Read the model definition and answer for the solid it produces. Units are mm, in the model's axes. Face numbers are marked on the shaded views. A direction names the side the tool comes from. Coordinates: 2 decimals unless noted, no trailing zeros. Order: outer loops, then holes, each group sorted by start corner. A loop starts at its lowest first (then second) coordinate and runs counter-clockwise, first axis right, second up. Notation, with made-up numbers: (49, 25.5) -> (55, 25.5) arc R30 cw to (55, 61.5) -> close; hole circle Ø9 at (-2, 42). An arc over 180 degrees is marked (long way). Answer as a JSON object with one key per item and string values. Group by question number.
1) Section D-D on z = -2 is taken. Determine the outline of the cut face in (x, y) (3 decimals).
2) Determine the mould class of the marked faces 1, 2 and 3 for opening direction Z: released by +Z, released by -Z, zero draft, split by the parting line, or undercut.
3) Given pin 1 (3.5 mm diameter, centred on x = 0, z = 0, fed in from -Y); pin 2 (3 mm diameter, centred on x = -1.5, y = 5.5, fed in from -Z); pin 3 (1 mm diameter, centred on x = 0, z = 0, fed in from +Y), each flat-ended and moving along its own axis, determine where each tip first touches the part or whether it passes through.
4) Section C-C on y = 4 is taken. Determine the outline of the cut face in (x, z), and give its area (3 significant figures).
5) Consider L1, parallel to Y at x = 0, z = -3.5 (3 decimals); L2, parallel to X at y = 5.5, z = 0.5; L3, parallel to Y at x = 0, z = 0. Determine where each line is inside the solid, lowest interval first.
6) Section A-A on z = 1 is taken. Determine the outline of the cut face in (x, y) (3 decimals), and give its area (3 significant figures).
7) A tool of negligible diameter and unlimited length cuts with its end or side. For the marked faces 4, 5 and 6, from which of +Z, -Z, +X, -X, +Y, -Y can it reach the whole face along a straight path? Write none if from no direction.
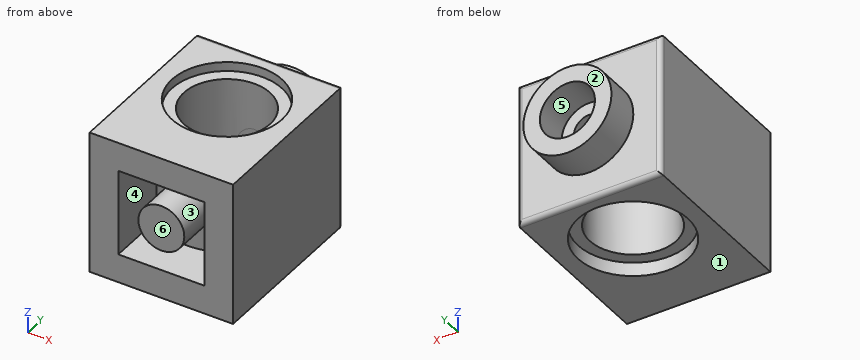
from build123d import *

# Parameters (mm, degrees)
SKETCH1_W                = 7.9375
SKETCH1_H                = 7.9375
BASE_EXTRUDE_DEPTH       = 9.525
SKETCH2_R                = 2.4384
BOSS_EXTRUDE1_DEPTH      = 1.905
SHELL1_T                 = -1.5875
SKETCH5_R                = 2.3876
CUT_EXTRUDE1_DEPTH       = 15.470652467
SKETCH6_R                = 3.048
CBORE1_DEPTH             = 0.508
CBORE2_START             = -0.762
SKETCH7_R                = 3.048
CBORE2_DEPTH             = 0.762
BOSS_EXTRUDE_THIN1_START = -5.842
SKETCH8_R                = 3.3876
SKETCH8_R_2              = 2.3876
BOSS_EXTRUDE_THIN1_DEPTH = 4.7625
INSDOT2_REACH            = 14.734
INSDOT2_END_RADIUS       = 3.3876
SKETCH4_R                = 1.27
CUT_EXTRUDE2_START       = -1.905
SKETCH10_R               = 1.524
CUT_EXTRUDE2_DEPTH       = 1.905
FILLET1_R                = 0.254


with BuildPart() as part:
    # Sketch1 → Base-Extrude (new body)
    with BuildSketch(Plane(origin=(0, 0, 0), x_dir=(1, 0, 0), z_dir=(0, 1, 0))):
        Rectangle(SKETCH1_W, SKETCH1_H)
    extrude(amount=BASE_EXTRUDE_DEPTH)

    # Sketch2 → Boss-Extrude1 (add)
    with BuildSketch(Plane(origin=(0, 9.525, 0), x_dir=(-1, 0, 0), z_dir=(0, 1, 0))):
        with Locations(Location((0, 0, 0), (0, 0, 270))):
            Circle(SKETCH2_R)
    extrude(amount=BOSS_EXTRUDE1_DEPTH)

    # Shell1
    shell1_openings = [part.faces().sort_by_distance(p)[0] for p in [
        (0, 0, 0),
    ]]
    offset(amount=SHELL1_T, openings=shell1_openings, kind=Kind.INTERSECTION)

    # Sketch5 → Cut-Extrude1 (cut, through all)
    with BuildSketch(Plane.XY.offset(3.96875)):
        with Locations((0, 5.715)):
            Circle(SKETCH5_R)
    extrude(amount=-CUT_EXTRUDE1_DEPTH, mode=Mode.SUBTRACT)

    # Sketch6 → cbore1 (cut)
    with BuildSketch(Plane.XY.offset(3.96875)):
        with Locations((0, 5.715)):
            Circle(SKETCH6_R)
    extrude(amount=-CBORE1_DEPTH, mode=Mode.SUBTRACT)

    # Sketch7 → cbore2 (cut)
    with BuildSketch(Plane(origin=(0, 0, -3.96875), x_dir=(-1, 0, 0), z_dir=(0, 0, -1)).offset(CBORE2_START)):
        with Locations(Location((0, 5.715, 0), (0, 0, 180))):
            Circle(SKETCH7_R)
    extrude(amount=CBORE2_DEPTH, mode=Mode.SUBTRACT)

    # Sketch8 → Boss-Extrude-Thin1 (add)
    with BuildSketch(Plane.XY.offset(3.46075).offset(BOSS_EXTRUDE_THIN1_START)):
        with Locations((0, 5.715)):
            Circle(SKETCH8_R)
        with Locations((0, 5.715)):
            Circle(SKETCH8_R_2, mode=Mode.SUBTRACT)
    extrude(amount=BOSS_EXTRUDE_THIN1_DEPTH)

    # InsDot2: up to this cylinder (the profile starts outside it)
    insdot2_end = Plane(origin=(0, 5.715, 0), z_dir=(0, 0, 1)) * Cylinder(INSDOT2_END_RADIUS, 37.2432, mode=Mode.PRIVATE)
    # Sketch4 → InsDot2 (add, up to the surface)
    with BuildSketch(Plane.XZ, mode=Mode.PRIVATE) as insdot2_sk1:
        with Locations(Location((0, 0, 0), (0, 0, 270))):
            Circle(SKETCH4_R)
    insdot2_tool1 = extrude(insdot2_sk1.sketch, amount=-INSDOT2_REACH, mode=Mode.PRIVATE) - insdot2_end
    add(insdot2_tool1.solids().sort_by_distance((0, 0, 0))[0])

    # Sketch10 → Cut-Extrude2 (cut)
    with BuildSketch(Plane(origin=(0, 11.43, 0), x_dir=(-1, 0, 0), z_dir=(0, 1, 0)).offset(CUT_EXTRUDE2_START)):
        with Locations(Location((0, 0, 0), (0, 0, 90))):
            Circle(SKETCH10_R)
    extrude(amount=CUT_EXTRUDE2_DEPTH, mode=Mode.SUBTRACT)

    # Fillet1
    fillet1_edges = [part.edges().sort_by_distance(p)[0] for p in [
        (3.96875, 9.525, 0),
        (0, 9.525, -3.96875),
        (-3.96875, 9.525, 0),
        (0, 9.525, 3.96875),
    ]]
    fillet(fillet1_edges, radius=FILLET1_R)


solid = part.part
Worked answers:
{
 "1": {"outline": "(-3.969, 0) -> (-2.381, 0) -> (-2.381, 3.306) arc R3.388 ccw to (2.381, 3.306) -> (2.381, 0) -> (3.969, 0) -> (3.969, 9.271) arc R0.254 ccw to (3.715, 9.525) -> (1.395, 9.525) -> (1.395, 11.43) -> (-1.395, 11.43) -> (-1.395, 9.525) -> (-3.715, 9.525) arc R0.254 ccw to (-3.969, 9.271) -> close; hole circle Ø4.775 at (0, 5.715)"},
 "2": {"face 1": "released by -Z", "face 2": "zero draft", "face 3": "undercut"},
 "3": {"pin 1": "stops at y = 0", "pin 2": "stops at z = -3.21", "pin 3": "stops at y = 9.1"},
 "4": {"outline": "(-3.97, -3.97) -> (-2.52, -3.97) -> (-2.52, -3.21) -> (-1.66, -3.21) -> (-1.66, 3.46) -> (-2.52, 3.46) -> (-2.52, 3.97) -> (-3.97, 3.97) -> close; (1.66, -3.21) -> (2.52, -3.21) -> (2.52, -3.97) -> (3.97, -3.97) -> (3.97, 3.97) -> (2.52, 3.97) -> (2.52, 3.46) -> (1.66, 3.46) -> close", "area": "34.5 mm²"},
 "5": {"L1": "y = 0 to 2.667, 8.763 to 9.525", "L2": "x = -3.97 to -2.38, 2.38 to 3.97", "L3": "y = 0 to 3.33, 8.1 to 9.1"},
 "6": {"outline": "(-3.969, 0) -> (-2.381, 0) -> (-2.381, 3.306) arc R3.388 ccw to (-0.783, 2.419) -> (-0.783, 0) -> (0.783, 0) -> (0.783, 2.419) arc R3.388 ccw to (2.381, 3.306) -> (2.381, 0) -> (3.969, 0) -> (3.969, 9.271) arc R0.254 ccw to (3.715, 9.525) -> (2.224, 9.525) -> (2.224, 11.43) -> (1.15, 11.43) -> (1.15, 9.525) -> (-1.15, 9.525) -> (-1.15, 11.43) -> (-2.224, 11.43) -> (-2.224, 9.525) -> (-3.715, 9.525) arc R0.254 ccw to (-3.969, 9.271) -> close; hole circle Ø4.775 at (0, 5.715)", "area": "52.9 mm²"},
 "7": {"face 4": "-Y", "face 5": "+Y", "face 6": "+Z, -Z, +X, -X, -Y"}
}
